Can you work these out from the model? Positions are in its coordinate system, mm. A direction names the side the tool comes from. Round coordinates to 2 decimals unless told otherwise and drop trailing zeros. Loops run counter-clockwise (first coordinate to the right, second up) from the corner with the lowest first, then second, coordinate; pieces in that order, holes last. Notation, with made-up numbers: (8.5, -36.5) -> (51.5, -36.5) arc R21 ccw to (51.5, 0.5) -> close; hole circle Ø3 at (69.5, -6.75). An arc over 180 degrees is marked (long way). Write each question's results on one line, items separated by ' | '.
from build123d import *

# Parameters (mm, degrees)
BOSS_EXTRUDE1_DEPTH = 10
BOSS_EXTRUDE2_START = 4
BOSS_EXTRUDE2_DEPTH = 4
FILLET1_R           = 1
FILLET2_R           = 3
FILLET3_R           = 1


with BuildPart() as part:
    # Sketch2 → Boss-Extrude1 (new body)
    with BuildSketch(Plane(origin=(0, 0, 0), x_dir=(1, 0, 0), z_dir=(0, 1, 0))):
        with BuildLine():
            Line((8.117655452, 42.627745196), (16.764304352, 34.685510469))
            ThreePointArc((16.764304352, 34.685510469), (18.147506186, 33.536916036), (19.638391538, 32.53203925))
            ThreePointArc((19.638391538, 32.53203925), (0, -38), (-19.638391538, 32.53203925))
            ThreePointArc((-19.638391538, 32.53203925), (-18.147506186, 33.536916036), (-16.764304352, 34.685510469))
            Line((-16.764304352, 34.685510469), (-8.117655452, 42.627745196))
            ThreePointArc((-8.117655452, 42.627745196), (0, 45.790117123), (8.117655452, 42.627745196))
        make_face()
        with BuildLine():
            Line((-6.764712877, 41.154807184), (-15.411361777, 33.212572457))
            ThreePointArc((-15.411361777, 33.212572457), (-16.948252704, 31.93635642), (-18.604791984, 30.819826658))
            ThreePointArc((-18.604791984, 30.819826658), (0, -36), (18.604791984, 30.819826658))
            ThreePointArc((18.604791984, 30.819826658), (16.948252704, 31.93635642), (15.411361777, 33.212572457))
            Line((15.411361777, 33.212572457), (6.764712877, 41.154807184))
            ThreePointArc((6.764712877, 41.154807184), (0, 43.790117123), (-6.764712877, 41.154807184))
        make_face(mode=Mode.SUBTRACT)
    extrude(amount=-BOSS_EXTRUDE1_DEPTH)

    # Sketch2<2> → Boss-Extrude2 (add)
    with BuildSketch(Plane(origin=(0, 0, 0), x_dir=(1, 0, 0), z_dir=(0, 1, 0)).offset(BOSS_EXTRUDE2_START)):
        with BuildLine():
            Line((8.117655452, 42.627745196), (16.764304352, 34.685510469))
            ThreePointArc((16.764304352, 34.685510469), (18.147506186, 33.536916036), (19.638391538, 32.53203925))
            ThreePointArc((19.638391538, 32.53203925), (0, -38), (-19.638391538, 32.53203925))
            ThreePointArc((-19.638391538, 32.53203925), (-18.147506186, 33.536916036), (-16.764304352, 34.685510469))
            Line((-16.764304352, 34.685510469), (-8.117655452, 42.627745196))
            ThreePointArc((-8.117655452, 42.627745196), (0, 45.790117123), (8.117655452, 42.627745196))
        make_face()
    extrude(amount=-BOSS_EXTRUDE2_DEPTH)

    # Fillet1
    fillet1_edges = [part.edges().sort_by_distance(p)[0] for p in [
        (16.948252704, 0, -31.93635642),
        (11.088037327, 0, -37.183689821),
        (0, 0, -43.790117123),
        (-11.088037327, 0, -37.183689821),
        (-16.948252704, 0, -31.93635642),
        (0, 0, 36),
    ]]
    fillet(fillet1_edges, radius=FILLET1_R)

    # Fillet2
    fillet2_edges = [part.edges().sort_by_distance(p)[0] for p in [
        (-18.147506186, 4, -33.536916036),
        (12.440979902, 4, -38.656627833),
        (0, 4, -45.790117123),
        (0, 4, 38),
        (18.147506186, 4, -33.536916036),
        (-12.440979902, 4, -38.656627833),
    ]]
    fillet(fillet2_edges, radius=FILLET2_R)

    # Fillet3
    fillet3_edges = [part.edges().sort_by_distance(p)[0] for p in [
        (18.147506186, -10, -33.536916036),
        (12.440979902, -10, -38.656627833),
        (0, -10, -45.790117123),
        (16.948252704, -10, -31.93635642),
        (0, -10, 36),
        (-16.948252704, -10, -31.93635642),
        (-11.088037327, -10, -37.183689821),
        (0, -10, -43.790117123),
        (11.088037327, -10, -37.183689821),
        (-12.440979902, -10, -38.656627833),
        (-18.147506186, -10, -33.536916036),
        (0, -10, 38),
    ]]
    fillet(fillet3_edges, radius=FILLET3_R - 0.0001)  # a hair under: the kernel refuses the full size


solid = part.part
1. We'd pull the mould along Z, two halves only. Please class faces 1 (the face through (1.382, -3.93, 37.975)), 2 (the face through (-1.309, -4.944, 35.976)), 3 (the face through (18.13, -3.93, -33.55)): pulls with the +Z half, pulls with the -Z half, needs draft (parallel to the pull), parting line crosses it, or undercut.
Final values:
face 1: parting line crosses it | face 2: undercut | face 3: pulls with the -Z half
2. On a 3-axis mill with a long thin cutter (end or side, diameter ignored), from which of +Z, -Z, +X, -X, +Y, -Y can I reach the whole of each face in a straight line? I mean faces 4 (the face through (0.1, -4.94, -43.79)), 5 (the face through (-18.2, -3.9, -33.5)). Say none if no direction works.
Final values:
face 4: -Y | face 5: -Z, -X, +Y, -Y
3. Will these pins go through, and if not, where does the flat tip stop? pin 1 (1.5 mm diameter, centred on x = 1, y = 2.5, fed in from -Z); pin 2 (6 mm diameter, centred on y = -4, z = 24, fed in from -X); pin 3 (2 mm diameter, centred on y = -8, z = 19, fed in from +X).
Final values:
pin 1: z = -45.66 | pin 2: x = -31.67 | pin 3: x = 33.47
4. If we section it at A-A (y = -3.25): List the corners of the cut face in (x, z) for me.
Final values:
outline: (-19.64, -32.53) arc R18 cw to (-16.76, -34.69) -> (-8.12, -42.63) arc R12 ccw to (8.12, -42.63) -> (16.76, -34.69) arc R18 cw to (19.64, -32.53) arc R38 ccw (long way) to start; hole (-18.6, -30.82) arc R20 cw to (-15.41, -33.21) -> (-6.76, -41.15) arc R10 ccw to (6.76, -41.15) -> (15.41, -33.21) arc R20 cw to (18.6, -30.82) arc R36 ccw (long way) to start
5. Please list where these lines run through material, in increasing order: line 1 (X direction, y = -5.75, z = 0); line 2 (X direction, y = -7.75, z = 29); line 3 (Y direction, x = 20.5, z = 1). Write a range as from..to.
Final values:
line 1: -38..-36, 36..38 | line 2: -24.56..-21.33, 21.33..24.56 | line 3: 0..4
